Verification items for the finished model (mm, model axes). A direction names the side the tool comes from. Round coordinates to 2 decimals unless told otherwise and drop trailing zeros. Order: outer loops, then holes, each group sorted by start corner. A loop starts at its lowest first (then second) coordinate and runs counter-clockwise, first axis right, second up. Notation, with made-up numbers: (78, 77.25) -> (88, 77.25) arc R24 ccw to (88, 89.25) -> close; hole circle Ø9 at (86.5, 46.25). An arc over 180 degrees is marked (long way). Answer in a Markdown table with one row per item. Add a question column.
```python
from build123d import *

# Parameters (mm, degrees)
SKETCH7_R             = 2.7
BOSS_EXTRUDE5_DEPTH   = 10
SKETCH7_W             = 22
SKETCH7_H             = 5
BOSS_EXTRUDE5_2_DEPTH = 10
SKETCH7_4_W           = 42
SKETCH7_4_H           = 10
SKETCH7_4_W_2         = 10
SKETCH7_4_H_2         = 5
SKETCH7_4_W_3         = 40
BOSS_EXTRUDE6_DEPTH   = 52
CUT_EXTRUDE3_REACH    = 58.502
SKETCH8_R             = 1.7


with BuildPart() as part:
    # Sketch7 → Boss-Extrude5 (new body)
    with BuildSketch(Plane.XY):
        Polygon((-65, -35), (-25, -35), (-25, -10), (-65, -10), (-65, -17.316919029), align=None)
        with Locations((-55, -22.5)):
            Circle(SKETCH7_R, mode=Mode.SUBTRACT)
        with Locations((-35, -22.5)):
            Circle(SKETCH7_R, mode=Mode.SUBTRACT)
    extrude(amount=BOSS_EXTRUDE5_DEPTH)



with BuildPart() as body_2:
    # Sketch7 → Boss-Extrude5 2 (new body)
    with BuildSketch(Plane.XY):
        with Locations((6, 2.5)):
            Rectangle(SKETCH7_W, SKETCH7_H)
    extrude(amount=BOSS_EXTRUDE5_2_DEPTH)


with BuildPart() as part_1:
    add(part.part)

    add(body_2.part)  # Boss-Extrude6 merges body 2
    # Sketch7_4 → Boss-Extrude6 (add)
    with BuildSketch(Plane.XY):
        with Locations((6, -46.501763528)):
            Rectangle(SKETCH7_4_W, SKETCH7_4_H)
        Polygon((-15, -35), (-23.528645833, -35), (-25, -35), (-25, -51.501763528), (-15, -51.501763528), (-15, -41.501763528), align=None)
        Polygon((-25, -35), (-23.528645833, -35), (-15, -35), (-15, 0), (-25, 0), (-25, -10), align=None)
        with Locations((-20, 2.5)):
            Rectangle(SKETCH7_4_W_2, SKETCH7_4_H_2)
        with Locations((-10, 2.5)):
            Rectangle(SKETCH7_4_W_2, SKETCH7_4_H_2)
        with Locations((22, 2.5)):
            Rectangle(SKETCH7_4_W_2, SKETCH7_4_H_2)
        with Locations((-45, -5)):
            Rectangle(SKETCH7_4_W_3, SKETCH7_4_H)
    extrude(amount=BOSS_EXTRUDE6_DEPTH)

    # Sketch8 → Cut-Extrude3 (cut, up to next)
    with BuildSketch(Plane(origin=(0, 5, 0), x_dir=(1, 0, 0), z_dir=(0, 1, 0)), mode=Mode.PRIVATE) as cut_extrude3_sk1:
        with Locations((22, -47)):
            Circle(SKETCH8_R)
    cut_extrude3_tool1 = extrude(cut_extrude3_sk1.sketch, amount=-CUT_EXTRUDE3_REACH, mode=Mode.PRIVATE) & part_1.part
    add(cut_extrude3_tool1.solids().sort_by_distance((22, 5, 47))[0], mode=Mode.SUBTRACT)
    # Sketch8 → Cut-Extrude3 (cut, up to next)
    with BuildSketch(Plane(origin=(0, 5, 0), x_dir=(1, 0, 0), z_dir=(0, 1, 0)), mode=Mode.PRIVATE) as cut_extrude3_sk2:
        with Locations((22.296850592, -16)):
            Circle(SKETCH8_R)
    cut_extrude3_tool2 = extrude(cut_extrude3_sk2.sketch, amount=-CUT_EXTRUDE3_REACH, mode=Mode.PRIVATE) & part_1.part
    add(cut_extrude3_tool2.solids().sort_by_distance((22.296851, 5, 16))[0], mode=Mode.SUBTRACT)
    # Sketch8 → Cut-Extrude3 (cut, up to next)
    with BuildSketch(Plane(origin=(0, 5, 0), x_dir=(1, 0, 0), z_dir=(0, 1, 0)), mode=Mode.PRIVATE) as cut_extrude3_sk3:
        with Locations((-9, -47)):
            Circle(SKETCH8_R)
    cut_extrude3_tool3 = extrude(cut_extrude3_sk3.sketch, amount=-CUT_EXTRUDE3_REACH, mode=Mode.PRIVATE) & part_1.part
    add(cut_extrude3_tool3.solids().sort_by_distance((-9, 5, 47))[0], mode=Mode.SUBTRACT)
    # Sketch8 → Cut-Extrude3 (cut, up to next)
    with BuildSketch(Plane(origin=(0, 5, 0), x_dir=(1, 0, 0), z_dir=(0, 1, 0)), mode=Mode.PRIVATE) as cut_extrude3_sk4:
        with Locations((-9, -16)):
            Circle(SKETCH8_R)
    cut_extrude3_tool4 = extrude(cut_extrude3_sk4.sketch, amount=-CUT_EXTRUDE3_REACH, mode=Mode.PRIVATE) & part_1.part
    add(cut_extrude3_tool4.solids().sort_by_distance((-9, 5, 16))[0], mode=Mode.SUBTRACT)


solid = part_1.part
```
1) Depth check by flat-ended pin: P1, Ø1, axis at y = -30, z = 27, coming from the -X side; P2, Ø3, axis at x = -39, z = 7.5, coming from the -Y side; P3, Ø5.5, axis at x = 2.5, y = 2, coming from the +Z side. Enter the tip coordinate at first touch or a pass-through.
2) Cross-section at A-A, the plane z = 47. Record the boundary of the cut face in (x, y).
3) Cross-section at B-B, the plane x = -9. Record the boundary of the cut face in (y, z).
4) Thickness scan on L1, parallel to Z at x = -9, y = 3.8; L2, parallel to X at y = 2, z = 45; L3, parallel to X at y = 1, z = 16. Record the ranges inside material, lowest first. Write a range as [from, to].
5) Draft check along Z on faces 6 (the face through (-15, -21, 26)), 7 (the face through (-19, -25, 52)), 8 (the face through (-9.37, 2.54, 48.66)), 9 (the face through (22.8, 2.5, 48.5)). Enter one of: +Z half, -Z half, draft (parallel to the pull), parting line (faces both ways), or undercut.
6) Cross-section at D-D, the plane z = 19.5. Record the boundary of the cut face in (x, y), and give its area (3 significant figures).
7) Tool access check on faces 1 (the face through (-10.7, 2.54, 15.93)), 2 (the face through (-45, 0, 26)), 3 (the face through (6, 3, 10)), 4 (the face through (-45, -10, 31)), 5 (the face through (-45, -35, 5)). Record the directions out of +Z, -Z, +X, -X, +Y, -Y that give a thin tool (end or side, any length) a straight path to the whole face; none if there is none.
8) Cross-section at C-C, the plane x = -55. Record the boundary of the cut face in (y, z), and give its area (3 significant figures).
Results below:
| question | item | result |
|---|---|---|
| 1 | P1 | x = -25 |
| 1 | P2 | y = -35 |
| 1 | P3 | z = 10 |
| 2 | outline | (-65, -10) -> (-25, -10) -> (-25, -51.5) -> (27, -51.5) -> (27, -41.5) -> (-15, -41.5) -> (-15, 0) -> (-10.7, 0) -> (-10.7, 5) -> (-25, 5) -> (-25, 0) -> (-65, 0) -> close; (-7.3, 0) -> (-5, 0) -> (-5, 5) -> (-7.3, 5) -> close; (17, 0) -> (20.3, 0) -> (20.3, 5) -> (17, 5) -> close; (23.7, 0) -> (27, 0) -> (27, 5) -> (23.7, 5) -> close |
| 3 | outline | (-51.5, 0) -> (-41.5, 0) -> (-41.5, 52) -> (-51.5, 52) -> close; (0, 0) -> (5, 0) -> (5, 14.3) -> (0, 14.3) -> close; (0, 17.7) -> (5, 17.7) -> (5, 45.3) -> (0, 45.3) -> close; (0, 48.7) -> (5, 48.7) -> (5, 52) -> (0, 52) -> close |
| 4 | L1 | [0, 14.3], [17.7, 45.3], [48.7, 52] |
| 4 | L2 | [-25, -5], [17, 27] |
| 4 | L3 | [-25, -10.7], [-7.3, -5], [17, 20.6], [24, 27] |
| 5 | face 6 | draft |
| 5 | face 7 | +Z half |
| 5 | face 8 | undercut |
| 5 | face 9 | undercut |
| 6 | outline | (-65, -10) -> (-25, -10) -> (-25, -51.5) -> (27, -51.5) -> (27, -41.5) -> (-15, -41.5) -> (-15, 0) -> (-5, 0) -> (-5, 5) -> (-25, 5) -> (-25, 0) -> (-65, 0) -> close; (17, 0) -> (27, 0) -> (27, 5) -> (17, 5) -> close |
| 6 | area | 1,490 mm² |
| 7 | face 1 | +Y |
| 7 | face 2 | +Z, -Z, -X, +Y |
| 7 | face 3 | +Z, +Y |
| 7 | face 4 | +Z, -X, -Y |
| 7 | face 5 | +Z, -Z, -X, -Y |
| 8 | outline | (-35, 0) -> (-25.2, 0) -> (-25.2, 10) -> (-35, 10) -> close; (-19.8, 0) -> (0, 0) -> (0, 52) -> (-10, 52) -> (-10, 10) -> (-19.8, 10) -> close |
| 8 | area | 716 mm² |
